from build123d import *

# Parameters (mm, degrees)
F1_DEPTH = 101.6
F2_R     = 12.7
F3_R     = 6.35
F4_DEPTH = 101.601
F5_W     = 20.32
F5_H     = 24.3607418369
F5_H_2   = 23.7557509671
F6_DEPTH = 50.8


with BuildPart() as f1:
    # F0 (on Front) → F1 (new body)
    with BuildSketch(Plane.XZ):
        with BuildLine():
            Line((3.81, 51.1735859583), (-3.81, 51.1735859583))
            Line((-3.81, 51.1735859583), (-3.81, -37.7264140417))
            ThreePointArc((-3.81, -37.7264140417), (0, -57.3049861203), (3.81, -37.7264140417))
            Line((3.81, -37.7264140417), (3.81, 51.1735859583))
        make_face()
    extrude(amount=F1_DEPTH)

    # F2
    f2_edges = [f1.edges().sort_by_distance(p)[0] for p in [
        (0, -101.6, 51.173586),
        (0, 0, 51.173586),
    ]]
    fillet(f2_edges, radius=F2_R)

    # F3 (on face) → F4 (cut, through all)
    with BuildSketch(Plane(origin=(0, 0, 0), x_dir=(-1, 0, 0), z_dir=(0, 1, 0))):
        with Locations((0, -47.1449861203)):
            Circle(F3_R)
    extrude(amount=-F4_DEPTH, mode=Mode.SUBTRACT)

    # F5 (on face) → F6 (cut, symmetric)
    with BuildSketch(Plane.YZ.offset(3.81)):
        with Locations((-71.12, -49.9067849601)):
            Rectangle(F5_W, F5_H)
        with Locations((-30.48, -49.6042895252)):
            Rectangle(F5_W, F5_H_2)
    extrude(amount=F6_DEPTH, both=True, mode=Mode.SUBTRACT)


solid = f1.part
Source: CAD feature listing. Evaluate the final solid. Frame: model axes, mm. A direction names the side the tool comes from. Round coordinates to 2 decimals unless told otherwise and drop trailing zeros. Loops run counter-clockwise (first coordinate to the right, second up) from the corner with the lowest first, then second, coordinate; pieces in that order, holes last. Notation, with made-up numbers: (-6.75, -19) - (24.25, -19) arc R22 ccw to (24.25, 15) - close; hole circle Ø2 at (-10, 25). An arc over 180 degrees is marked (long way). Write item = value, one per line. Start each with the question number.
(1) Section query C-C, the plane z = 34.5. Output: boundary loops of the cut face in (x, y).
(2) Section query B-B, the plane y = -32. Output: boundary loops of the cut face in (x, z).
(3) Section query A-A, the plane x = 0. Output: boundary loops of the cut face in (y, z).
(4) Ray query, line 1 along Y through (x, z) = (3, -41); line 2 along Z through (x, y) = (0, -45.5); line 3 along X through (y, z) = (-22.5, -0.5). Return the intervals inside material, ascending. Write a range as from..to.
(5) Set-up query: faces 5 (the face through (-0.392, -50.658, -57.297)), 6 (the face through (3.81, -50, 6)), 7 (the face through (-4.4, -20.32, -52)), 8 (the face through (-3.81, -50, 7)), 9 (the face through (0, 0, -9)). Return all of +Z, -Z, +X, -X, +Y, -Y with unobstructed straight access to the full face (end or side cutting, diameter ignored); none if empty.
(6) Pin query (flat end, axial travel): pin 1 (7.5 mm diameter, centred on x = 0, z = -47.14, fed in from +Y); pin 2 (10 mm diameter, centred on y = -29.5, z = 28.5, fed in from +X); pin 3 (6 mm diameter, centred on x = -0.5, y = -71.5, fed in from -Z). Return the tip coordinate at first contact, or that it passes through.
(7) Pull-direction query (Z, two-part tool) for faces 1 (the face through (-0.053, -97.781, 47.552)), 2 (the face through (1.377, -91.298, -53.344)), 3 (the face through (1.377, -50.658, -53.344)), 4 (the face through (-0.392, -10.018, -57.297)); classes: +Z half, -Z half, draft (parallel to the pull), parting line (faces both ways), or undercut.
Conclusion:
q1.outline = (-3.81, -101.6) - (3.81, -101.6) - (3.81, 0) - (-3.81, 0) - close
q2.outline = (-3.81, -37.73) - (3.81, -37.73) - (3.81, 51.17) - (-3.81, 51.17) - close
q3.outline = (-101.6, -57.3) - (-81.28, -57.3) - (-81.28, -53.49) - (-101.6, -53.49) - close; (-101.6, -40.79) - (-81.28, -40.79) - (-81.28, -37.73) - (-60.96, -37.73) - (-60.96, -40.79) - (-40.64, -40.79) - (-40.64, -37.73) - (-20.32, -37.73) - (-20.32, -40.79) - (0, -40.79) - (0, 38.47) arc R12.7 ccw to (-12.7, 51.17) - (-88.9, 51.17) arc R12.7 ccw to (-101.6, 38.47) - close; (-60.96, -57.3) - (-40.64, -57.3) - (-40.64, -53.49) - (-60.96, -53.49) - close; (-20.32, -57.3) - (0, -57.3) - (0, -53.49) - (-20.32, -53.49) - close
q4.line_1 = -101.6..-81.28, -60.96..-40.64, -20.32..0
q4.line_2 = -57.3..-53.49, -40.79..51.17
q4.line_3 = -3.81..3.81
q5.face_5 = +Y, -Y
q5.face_6 = +Z, +X, +Y, -Y
q5.face_7 = -Z, +X, -X
q5.face_8 = +Z, -X, +Y, -Y
q5.face_9 = +Z, -Z, +X, -X, +Y
q6.pin_1 = through
q6.pin_2 = 3.81
q6.pin_3 = -37.73
q7.face_1 = +Z half
q7.face_2 = undercut
q7.face_3 = undercut
q7.face_4 = parting line
